Here's how the part is built. I have some questions about the finished solid (model axes, mm). A direction names the side the tool comes from. Give positions to 0.01 mm unless a question says otherwise; leave off trailing zeros. Write each loop counter-clockwise with the first axis right and the second up, starting at its lowest first coordinate (ties: lowest second). Pieces come first, ordered by that corner, then holes. Notation, with made-up numbers: M 36,32.5 L 83,32.5 A15 ccw 83,53.5 Z; hole C 35,18 d4. An arc over 180 degrees is marked long. Answer as CSV lines item,"result". Start each with the question number.
Q1. Suppose I cut it at D-D (y = -25.4). Write out the boundary of the cut face in (x, z).
Q2. Suppose I cut it at B-B (y = -36). Write out the boundary of the cut face in (x, z).
Q3. On a 3-axis mill with a long thin cutter (end or side, diameter ignored), from which of +Z, -Z, +X, -X, +Y, -Y can I reach the whole of each face in a straight line? I mean faces 1 (the flat face through (-1, -50.8, -7)), 2 (the flat face through (0, -48, 10.16)), 3 (the flat face through (-45.72, -26, 8)). Say none if no direction works.
Q4. For pin 1 (6 mm diameter, centred on x = 36.5, z = 5.5, fed in from +Y); pin 2 (2.5 mm diameter, centred on x = 6, y = -47.5, fed in from +Z); pin 3 (10 mm diameter, centred on y = -25.4, z = 0, fed in from +X), each with a flat end and sliding along its axis, tell me the tip position at first contact or that it passes through.
Q5. Thinking about a two-plate mould opening in X: for faces 4 (the flat face through (-1, -45.72, -7)), 5 (the flat face through (50.8, -25, 7)), 6 (the cylindrical face through (-48.224, -19.343, 1.907)), which applies, +X half, -X half, draft (parallel to the pull), parting line (faces both ways), or undercut?
Q6. Suppose I cut it at C-C (x = -17.5). Write out the boundary of the cut face in (y, z).
Q7. Suppose I cut it at A-A (z = 0). Write out the boundary of the cut face in (x, y), then the cut area to 3 significant figures.
Q8. If I drill on line 1 along Y through (x, z) = (19.5, 6.5); line 2 along X through (y, z) = (-33.5, -17.5); line 3 along Z through (x, y) = (-48, -25.4), over which ranges is the centre line in solid material (lowest first)?
```python
from build123d import *

# Parameters (mm, degrees)
F0_W     = 101.6
F0_H     = 63.5
F1_DEPTH = 50.8
F2_W     = 50.8
F2_H     = 21.59
F3_DEPTH = 70.866
F4_W     = 91.44
F4_H     = 40.64
F5_DEPTH = 71.628
F6_R     = 6.35
F7_DEPTH = 111.506


with BuildPart() as f1:
    # F0 (on Front) → F1 (new body)
    with BuildSketch(Plane.XZ):
        Rectangle(F0_W, F0_H)
    extrude(amount=F1_DEPTH)

    # F2 (on face) → F3 (cut)
    with BuildSketch(Plane.XZ.offset(50.8)):
        with Locations((0, 20.955)):
            Rectangle(F2_W, F2_H)
    extrude(amount=-F3_DEPTH, mode=Mode.SUBTRACT)

    # F4 (on face) → F5 (cut)
    with BuildSketch(Plane.XY.offset(31.75)):
        with Locations((0, -25.4)):
            Rectangle(F4_W, F4_H)
    extrude(amount=-F5_DEPTH, mode=Mode.SUBTRACT)

    # F6 (on face) → F7 (cut)
    with BuildSketch(Plane.YZ.offset(50.8)):
        with Locations((-25.4, 0)):
            Circle(F6_R)
    extrude(amount=-F7_DEPTH, mode=Mode.SUBTRACT)


solid = f1.part
```
Resolved:
1,outline,"M -50.8,-31.75 L -45.72,-31.75 L -45.72,-6.35 L -50.8,-6.35 Z; M -50.8,6.35 L -45.72,6.35 L -45.72,31.75 L -50.8,31.75 Z; M 45.72,-31.75 L 50.8,-31.75 L 50.8,-6.35 L 45.72,-6.35 Z; M 45.72,6.35 L 50.8,6.35 L 50.8,31.75 L 45.72,31.75 Z"
2,outline,"M -50.8,-31.75 L -45.72,-31.75 L -45.72,31.75 L -50.8,31.75 Z; M 45.72,-31.75 L 50.8,-31.75 L 50.8,31.75 L 45.72,31.75 Z"
3,face 1,"+Z, -Z, +X, -X, -Y"
3,face 2,"+Z, +Y, -Y"
3,face 3,"+Z, -Z"
4,pin 1,"y = 0"
4,pin 2,"z = 10.16"
4,pin 3,"through"
5,face 4,"undercut"
5,face 5,"+X half"
5,face 6,"draft"
6,outline,"M -50.8,-31.75 L -45.72,-31.75 L -45.72,10.16 L -50.8,10.16 Z; M -5.08,-31.75 L 0,-31.75 L 0,10.16 L -5.08,10.16 Z"
7,outline,"M -50.8,-50.8 L 50.8,-50.8 L 50.8,-31.75 L 45.72,-31.75 L 45.72,-45.72 L -45.72,-45.72 L -45.72,-31.75 L -50.8,-31.75 Z; M -50.8,-19.05 L -45.72,-19.05 L -45.72,-5.08 L 45.72,-5.08 L 45.72,-19.05 L 50.8,-19.05 L 50.8,0 L -50.8,0 Z"
7,area,"1,320 mm^2"
8,line 1,"-50.8 to -45.72, -5.08 to 0"
8,line 2,"-50.8 to -45.72, 45.72 to 50.8"
8,line 3,"-31.75 to -6.35, 6.35 to 31.75"
